Source: CAD feature listing. Evaluate the final solid. Frame: model axes, mm. Face numbers are marked on the shaded views. Round coordinates to 2 decimals unless told otherwise and drop trailing zeros. Order: outer loops, then holes, each group sorted by start corner. A loop starts at its lowest first (then second) coordinate and runs counter-clockwise, first axis right, second up. Notation, with made-up numbers: (46, 79) -> (59, 79) arc R8 cw to (59, 94) -> close; hole circle Ø10 at (38.25, 32.5). An arc over 180 degrees is marked (long way). One line per item, written item: value. Start each with the question number.
1) Mould query, pull axis Y, two halves, no side actions, for the marked faces 1, 2 and 3. Classes: pulls with the +Y half, pulls with the -Y half, needs draft (parallel to the pull), parting line crosses it, or undercut.
2) Pin query (flat end, axial travel): P1, Ø0.9, axis at y = 6.5, z = 28.5, coming from the -X side; P2, Ø2, axis at x = 6, z = 25.5, coming from the +Y side; P3, Ø17, axis at x = 28.5, z = 19.5, coming from the -Y side; P4, Ø5, axis at x = 15.5, z = 26, coming from the -Y side. Return the tip coordinate at first contact, or that it passes through.
3) Ray query, L1, parallel to Y at x = 14, z = 44; L2, parallel to X at y = 7, z = 24.5; L3, parallel to X at y = 0.75, z = 16. Return the intervals inside material, ascending.
4) Section C-C (x = 6.5). Return the cut outline in (y, z).
5) Section A-A (y = 2.75). Return the cut outline in (x, z), and give its area (3 significant figures).
6) Section D-D (y = 6.75). Return the cut outline in (x, z), and give its area (3 significant figures).
7) Section B-B (z = 21). Return the cut outline in (x, y).
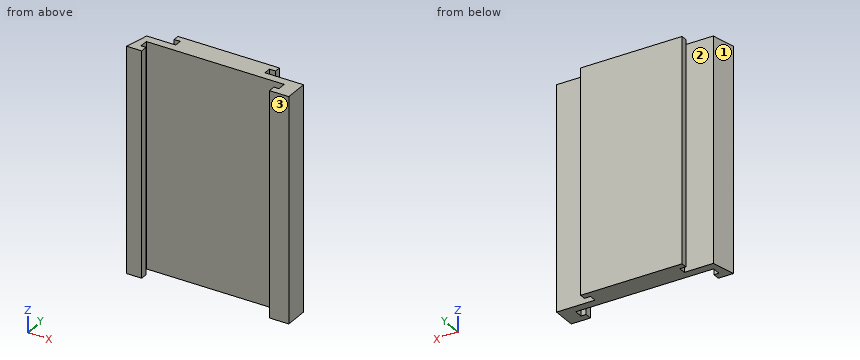
```python
from build123d import *

# Parameters (mm, degrees)
BOSS_EXTRUDE1_DEPTH = 55
CUT_EXTRUDE2_REACH  = 57


with BuildPart() as part:
    # Sketch2 → Boss-Extrude1 (new body)
    with BuildSketch(Plane.XY):
        Polygon((0, 0), (0, 5.85), (9.5, 5.85), (9.5, 7.65), (8, 7.65), (8, 9.15), (33, 9.15), (33, 7.65), (31.5, 7.65), (31.5, 5.85), (41, 5.85), (41, 0), (36.25, 0), (36.25, 1.75), (37.5, 1.75), (37.5, 3.85), (3.5, 3.85), (3.5, 1.75), (4.75, 1.75), (4.75, 0), align=None)
    extrude(amount=BOSS_EXTRUDE1_DEPTH)

    # Sketch3 → Cut-Extrude2 (cut, up to next)
    with BuildSketch(Plane.XY.offset(55), mode=Mode.PRIVATE) as cut_extrude2_sk1:
        Polygon((1, 0), (0, 0), (0, 5.85), (2.358395181, 5.85), align=None)
    cut_extrude2_tool1 = extrude(cut_extrude2_sk1.sketch, amount=-CUT_EXTRUDE2_REACH, mode=Mode.PRIVATE) & part.part
    add(cut_extrude2_tool1.solids().sort_by_distance((0.885385, 3.319366, 55))[0], mode=Mode.SUBTRACT)


solid = part.part
```
Findings:
1. face 1: pulls with the +Y half
1. face 2: undercut
1. face 3: pulls with the -Y half
2. P1: x = 9.5
2. P2: y = 5.85
2. P3: y = 0
2. P4: y = 3.85
3. L1: 3.85 to 9.15
3. L2: 9.5 to 31.5
3. L3: 1.17 to 4.75, 36.25 to 41
4. outline: (3.85, 0) -> (5.85, 0) -> (5.85, 55) -> (3.85, 55) -> close
5. outline: (1.64, 0) -> (3.5, 0) -> (3.5, 55) -> (1.64, 55) -> close; (37.5, 0) -> (41, 0) -> (41, 55) -> (37.5, 55) -> close
5. area: 295 mm2
6. outline: (9.5, 0) -> (31.5, 0) -> (31.5, 55) -> (9.5, 55) -> close
6. area: 1,210 mm2
7. outline: (1, 0) -> (4.75, 0) -> (4.75, 1.75) -> (3.5, 1.75) -> (3.5, 3.85) -> (37.5, 3.85) -> (37.5, 1.75) -> (36.25, 1.75) -> (36.25, 0) -> (41, 0) -> (41, 5.85) -> (31.5, 5.85) -> (31.5, 7.65) -> (33, 7.65) -> (33, 9.15) -> (8, 9.15) -> (8, 7.65) -> (9.5, 7.65) -> (9.5, 5.85) -> (2.36, 5.85) -> close
